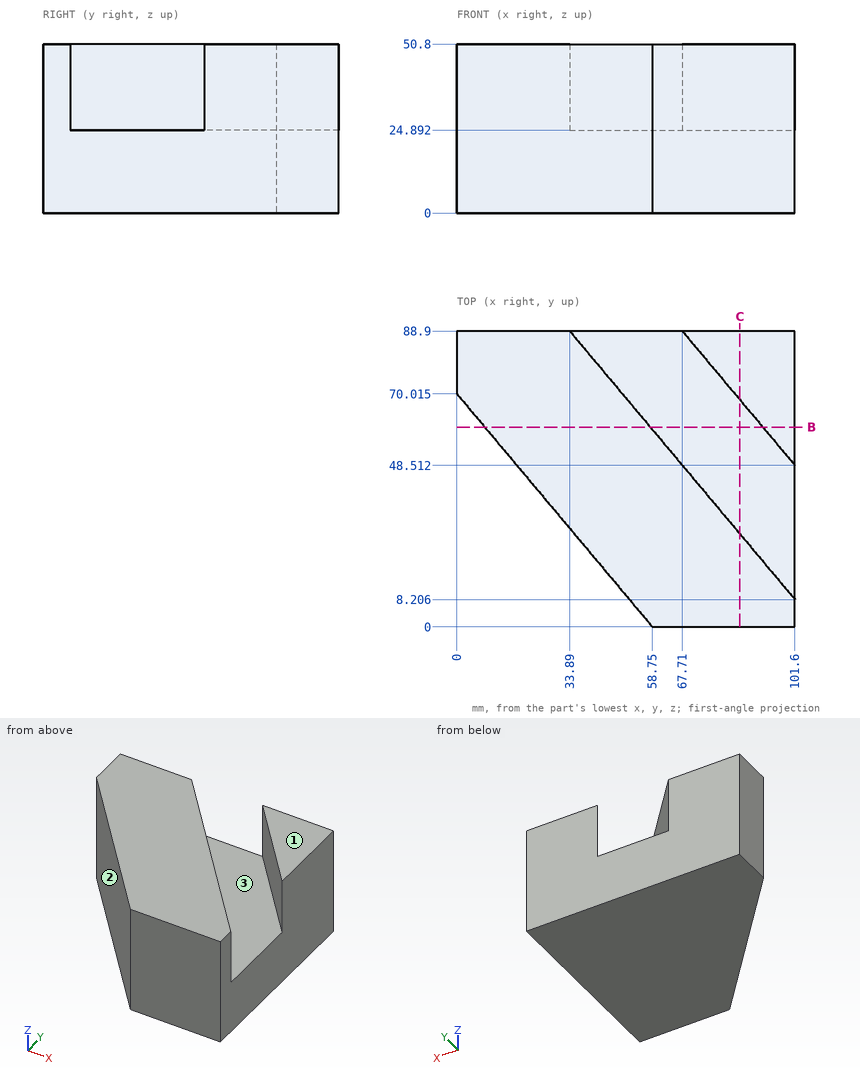
Study the drawing (mm; zero at the part's minimum x, y, z) and answer. Coordinates: 2 decimals unless noted, no trailing zeros. Loops run counter-clockwise (first coordinate to the right, second up) from the corner with the lowest first, then second, coordinate; pieces in that order, holes last. Notation, with made-up numbers: (46, 47.25) -> (84, 47.25) arc R16 cw to (84, 72.25) -> close; hole circle Ø10 at (20.5, 53). An arc over 180 degrees is marked (long way). Answer as CSV lines item,"result".
1) For a pull along Y with two mould halves and no side action, classify the marked faces 1, 2 and 3 as released by +Y, released by -Y, zero draft, split by the parting line, or undercut.
A:
face 1,"zero draft"
face 2,"released by -Y"
face 3,"undercut"
2) The part is cut by section B-B (y = 60). Give the vertices of the cut face in (x, z), and give its area (3 significant figures).
A:
outline,"(8.4, 0) -> (101.6, 0) -> (101.6, 50.8) -> (91.96, 50.8) -> (91.96, 24.89) -> (58.14, 24.89) -> (58.14, 50.8) -> (8.4, 50.8) -> close"
area,"3,860 mm²"
3) The part is cut by section C-C (x = 85). Give the vertices of the cut face in (y, z) (1 decimal), and give its area (3 significant figures).
A:
outline,"(0, 0) -> (88.9, 0) -> (88.9, 50.8) -> (68.3, 50.8) -> (68.3, 24.9) -> (28, 24.9) -> (28, 50.8) -> (0, 50.8) -> close"
area,"3,470 mm²"
4) Flat-ended cylindrical pins translate along their axes: pin 1 (3 mm diameter, centred on y = 18.5, z = 39.5, fed in from -X); pin 2 (12 mm diameter, centred on x = 29.5, z = 27, fed in from -Y); pin 3 (3 mm diameter, centred on y = 13, z = 42.5, fed in from -X). Find the tip coordinate at first contact, or state that the pin passes through.
A:
pin 1,"stops at x = 41.97"
pin 2,"stops at y = 27.71"
pin 3,"stops at x = 46.58"
5) Straight lines are drawn through the part: probe 1 along Z at (x, y) = (76.5, 38.5); probe 2 along X at (y, z) = (59.5, 28); probe 3 along Y at (x, z) = (96, 34.5) (1 decimal). For each, find the intervals that lie inside material, in ascending order.
A:
probe 1,"z = 0 to 24.89"
probe 2,"x = 8.82 to 58.56, 92.38 to 101.6"
probe 3,"y = 0 to 14.9, 55.2 to 88.9"
